Source: three-view drawing plus pictorial views. Frame: mm from the lowest corner of the part. Give positions to 0.01 mm unless a question says otherwise; leave off trailing zeros. Order: outer loops, then holes, each group sorted by start corner. A loop starts at its lowest first (then second) coordinate and runs counter-clockwise, first axis right, second up. Notation, with made-up numbers: (56, 18.25) -> (93, 18.25) arc R22 ccw to (93, 25.25) -> close; hole circle Ø10 at (-36, -2). An arc over 180 degrees is marked (long way). Answer in a Markdown table with one row per item. Add a question column.
Q1. Cut plane C-C on z = 1.15. Return the cut outline in (x, y), and give its area (3 significant figures).
Q2. Cut plane A-A on x = 13. Return the cut outline in (y, z).
Q3. Line query: line 1 along Y through (x, z) = (2.75, 1.1); line 2 along Y through (x, z) = (23.5, 0.6); line 3 along X through (y, z) = (23.5, 0.65). Output: solid intervals per line, ascending. Write a range as from..to.
Q4. Cut plane D-D on y = 2. Return the cut outline in (x, z), and give its area (3 significant figures).
Q5. Cut plane B-B on y = 7. Return the cut outline in (x, z).
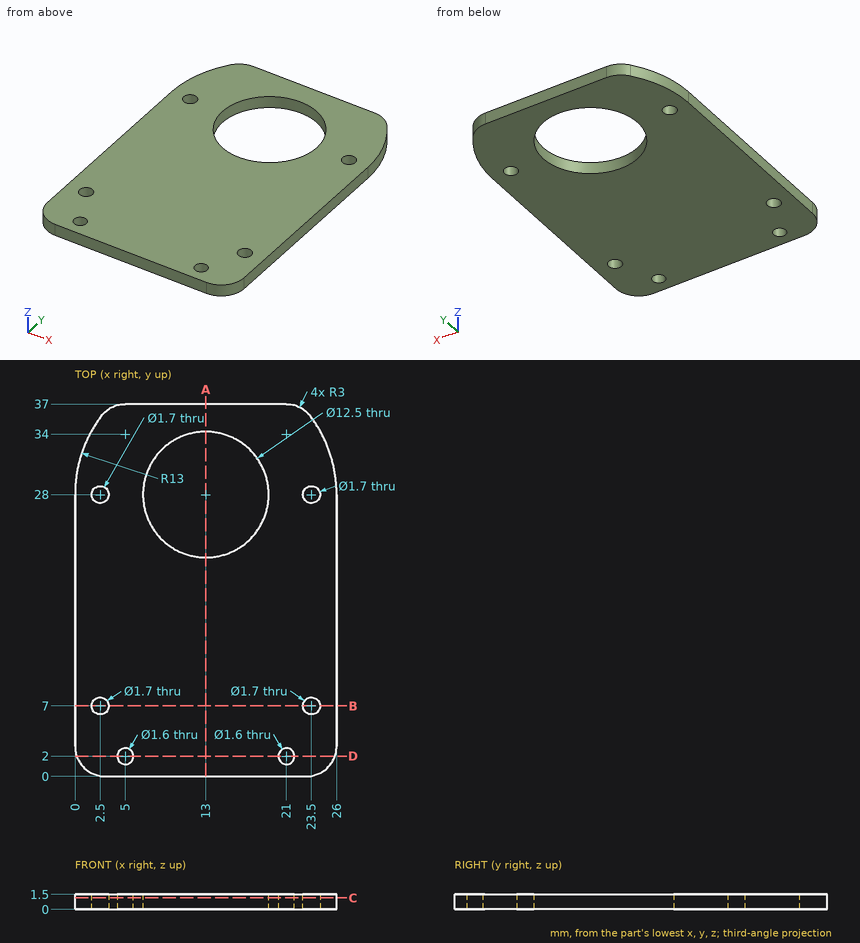
Completed:
| question | item | result |
|---|---|---|
| 1 | outline | (0, 3) arc R3 ccw to (3, 0) -> (23, 0) arc R3 ccw to (26, 3) -> (26, 28) arc R13 ccw to (23.4, 35.8) arc R3 ccw to (21, 37) -> (5, 37) arc R3 ccw to (2.6, 35.8) arc R13 ccw to (0, 28) -> close; hole circle Ø1.7 at (2.5, 7); hole circle Ø1.7 at (2.5, 28); hole circle Ø1.6 at (5, 2); hole circle Ø12.5 at (13, 28); hole circle Ø1.6 at (21, 2); hole circle Ø1.7 at (23.5, 7); hole circle Ø1.7 at (23.5, 28) |
| 1 | area | 801 mm² |
| 2 | outline | (0, 0) -> (21.75, 0) -> (21.75, 1.5) -> (0, 1.5) -> close; (34.25, 0) -> (37, 0) -> (37, 1.5) -> (34.25, 1.5) -> close |
| 3 | line 1 | y = 0.01..6.19, 7.81..27.19, 28.81..35.98 |
| 3 | line 2 | y = 0.04..6.15, 7.85..27.15, 28.85..35.66 |
| 3 | line 3 | x = 0..8.66, 17.34..26 |
| 4 | outline | (0.17, 0) -> (4.2, 0) -> (4.2, 1.5) -> (0.17, 1.5) -> close; (5.8, 0) -> (20.2, 0) -> (20.2, 1.5) -> (5.8, 1.5) -> close; (21.8, 0) -> (25.83, 0) -> (25.83, 1.5) -> (21.8, 1.5) -> close |
| 4 | area | 33.7 mm² |
| 5 | outline | (0, 0) -> (1.65, 0) -> (1.65, 1.5) -> (0, 1.5) -> close; (3.35, 0) -> (22.65, 0) -> (22.65, 1.5) -> (3.35, 1.5) -> close; (24.35, 0) -> (26, 0) -> (26, 1.5) -> (24.35, 1.5) -> close |
